```python
from build123d import *

# Parameters (mm, degrees)
SKETCH1_R               = 13
BOSS_EXTRUDE1_DEPTH     = 2.5
BOSS_EXTRUDE2_START     = 2.5
SKETCH2_R               = 13
SKETCH2_R_2             = 11.5
BOSS_EXTRUDE2_DEPTH     = 15
CUT_EXTRUDE1_START      = 2.5
SKETCH3_R               = 5.5
CUT_EXTRUDE1_DEPTH      = 1.2
CUT_EXTRUDE2_DEPTH      = 26.382080293
CUT_EXTRUDE2_DEPTH_BACK = 26.382080293
SKETCH4_R               = 1.2
SKETCH4_R_2             = 2
SKETCH5_R               = 1.2
BOSS_EXTRUDE3_DEPTH     = 2.5


with BuildPart() as part:
    # Sketch1 → Boss-Extrude1 (new body)
    with BuildSketch(Plane(origin=(0, 0, 0), x_dir=(1, 0, 0), z_dir=(0, 1, 0))):
        with Locations(Location((0, 0, 0), (0, 0, 270))):
            Circle(SKETCH1_R)
    extrude(amount=BOSS_EXTRUDE1_DEPTH)

    # Sketch2 → Boss-Extrude2 (add)
    with BuildSketch(Plane(origin=(0, 0, 0), x_dir=(1, 0, 0), z_dir=(0, 1, 0)).offset(BOSS_EXTRUDE2_START)):
        with Locations(Location((0, 0, 0), (0, 0, 270))):
            Circle(SKETCH2_R)
        with Locations(Location((0, 0, 0), (0, 0, 270))):
            Circle(SKETCH2_R_2, mode=Mode.SUBTRACT)
    extrude(amount=BOSS_EXTRUDE2_DEPTH)

    # Sketch3 → Cut-Extrude1 (cut)
    with BuildSketch(Plane(origin=(0, 0, 0), x_dir=(1, 0, 0), z_dir=(0, 1, 0)).offset(CUT_EXTRUDE1_START)):
        with Locations(Location((0, 0, 0), (0, 0, 270))):
            Circle(SKETCH3_R)
    extrude(amount=-CUT_EXTRUDE1_DEPTH, mode=Mode.SUBTRACT)

    # Sketch4 → Cut-Extrude2 (cut, two sides: drawn at the far end of the back side and taken through both)
    with BuildSketch(Plane(origin=(0, 0, 0), x_dir=(1, 0, 0), z_dir=(0, 1, 0)).offset(-CUT_EXTRUDE2_DEPTH_BACK)):
        with Locations(Location((0, 8.5, 0), (0, 0, 270))):
            Circle(SKETCH4_R)
        with Locations(Location((7.361215932, -4.25, 0), (0, 0, 270))):
            Circle(SKETCH4_R)
        with Locations(Location((-7.361215932, -4.25, 0), (0, 0, 270))):
            Circle(SKETCH4_R)
        with Locations(Location((0, 0, 0), (0, 0, 270))):
            Circle(SKETCH4_R_2)
    extrude(amount=CUT_EXTRUDE2_DEPTH + CUT_EXTRUDE2_DEPTH_BACK, mode=Mode.SUBTRACT)

    # Sketch5 → Boss-Extrude3 (add)
    # profile 1 of 2: a face of its own
    with BuildSketch(Plane(origin=(0, 0, 0), x_dir=(1, 0, 0), z_dir=(0, 1, 0))):
        with BuildLine():
            Line((-3, 12.649110641), (-3, 16))
            ThreePointArc((-3, 16), (-2.121320344, 18.121320344), (0, 19))
            ThreePointArc((0, 19), (2.121320344, 18.121320344), (3, 16))
            Line((3, 16), (3, 12.649110641))
            ThreePointArc((3, 12.649110641), (0, 13), (-3, 12.649110641))
        make_face()
        with Locations(Location((0, 16, 0), (0, 0, 270))):
            Circle(SKETCH5_R, mode=Mode.SUBTRACT)
    # profile 2 of 2: a face of its own
    with BuildSketch(Plane(origin=(0, 0, 0), x_dir=(1, 0, 0), z_dir=(0, 1, 0))):
        with BuildLine():
            Line((3, -16), (3, -12.649110641))
            ThreePointArc((3, -12.649110641), (0, -13), (-3, -12.649110641))
            Line((-3, -12.649110641), (-3, -16))
            ThreePointArc((-3, -16), (-2.121320344, -18.121320344), (0, -19))
            ThreePointArc((0, -19), (2.121320344, -18.121320344), (3, -16))
        make_face()
        with Locations(Location((0, -16, 0), (0, 0, 90))):
            Circle(SKETCH5_R, mode=Mode.SUBTRACT)
    extrude(amount=BOSS_EXTRUDE3_DEPTH)


solid = part.part
```
Geometry check sheet. Reference: the model listing, model coordinates, mm. A direction names the side the tool comes from. Coordinates: 2 decimals unless noted, no trailing zeros. Order: outer loops, then holes, each group sorted by start corner. A loop starts at its lowest first (then second) coordinate and runs counter-clockwise, first axis right, second up. Notation, with made-up numbers: (69.5, -32.75) - (97.5, -32.75) arc R36 cw to (97.5, 6.25) - close; hole circle Ø8 at (56, 4). An arc over 180 degrees is marked (long way). Use one line per item in the form item = value.
1. Section check C-C (x = -10.25). Record the boundary of the cut face in (y, z), then the cut area to 3 significant figures.
Here are the results:
outline = (0, -8) - (17.5, -8) - (17.5, -5.21) - (2.5, -5.21) - (2.5, 5.21) - (17.5, 5.21) - (17.5, 8) - (0, 8) - close
area = 123 mm²
2. Access from +Z, -Z, +X, -X, +Y, -Y to the whole of each face (thin tool, end or side, straight path). Record for faces 4 (the face through (-3, 1, -14)), 5 (the face through (9.7, 9.9, 6.18)), 6 (the face through (-3, 1, 14)), 7 (the face through (3, 1, 14)).
Here are the results:
face_4 = -Z, -X, +Y, -Y
face_5 = +Y
face_6 = +Z, -X, +Y, -Y
face_7 = +Z, +X, +Y, -Y
3. Section check A-A (z = -8.5). Record the boundary of the cut face in (x, y).
Here are the results:
outline = (-9.84, 0) - (-1.2, 0) - (-1.2, 2.5) - (-7.75, 2.5) - (-7.75, 17.5) - (-9.84, 17.5) - close; (1.2, 0) - (9.84, 0) - (9.84, 17.5) - (7.75, 17.5) - (7.75, 2.5) - (1.2, 2.5) - close
4. Gauge pin test, flat ends, axial feed: pin 1 (2 mm diameter, centred on y = 2, z = 15, fed in from -X); pin 2 (5 mm diameter, centred on x = 0, z = -17.5, fed in from +Y); pin 3 (2 mm diameter, centred on x = 7.36, z = 4.25, fed in from +Y); pin 4 (3.5 mm diameter, centred on x = 2, z = 2.5, fed in from +Y). Record the tip position at first contact, or that the pin passes through.
Here are the results:
pin_1 = -3
pin_2 = 2.5
pin_3 = through
pin_4 = 1.3
5. Scan lines: line 1 (X direction, y = 0.8, z = 0); line 2 (X direction, y = 1, z = 4.25); line 3 (X direction, y = 2.2, z = 0). Record each from-to range of solid material in increasing order.
Here are the results:
line_1 = -13 to -2, 2 to 13
line_2 = -12.29 to -8.56, -6.16 to 6.16, 8.56 to 12.29
line_3 = -13 to -5.5, 5.5 to 13
6. Section check D-D (z = 4.25). Record the boundary of the cut face in (x, y).
Here are the results:
outline = (-12.29, 0) - (-8.56, 0) - (-8.56, 2.5) - (-10.69, 2.5) - (-10.69, 17.5) - (-12.29, 17.5) - close; (-6.16, 0) - (6.16, 0) - (6.16, 2.5) - (3.49, 2.5) - (3.49, 1.3) - (-3.49, 1.3) - (-3.49, 2.5) - (-6.16, 2.5) - close; (8.56, 0) - (12.29, 0) - (12.29, 17.5) - (10.69, 17.5) - (10.69, 2.5) - (8.56, 2.5) - close
7. Section check B-B (x = 6.75). Record the boundary of the cut face in (y, z), then the cut area to 3 significant figures.
Here are the results:
outline = (0, -11.11) - (17.5, -11.11) - (17.5, -9.31) - (2.5, -9.31) - (2.5, 3.22) - (0, 3.22) - close; (0, 5.28) - (2.5, 5.28) - (2.5, 9.31) - (17.5, 9.31) - (17.5, 11.11) - (0, 11.11) - close
area = 104 mm²
8. Draft check along Z on faces 1 (the face through (0.05, 1.23, -17.2)), 2 (the face through (3, 1, -14)), 3 (the face through (3.9, 8.6, 12.4)). Enter one of: pulls with the +Z half, pulls with the -Z half, needs draft (parallel to the pull), parting line crosses it, or undercut.
Here are the results:
face_1 = undercut
face_2 = needs draft
face_3 = parting line crosses it
